Read the model definition and answer for the solid it produces. Units are mm, in the model's axes. A direction names the side the tool comes from. Round coordinates to 2 decimals unless told otherwise and drop trailing zeros. Loops run counter-clockwise (first coordinate to the right, second up) from the corner with the lowest first, then second, coordinate; pieces in that order, holes last. Notation, with made-up numbers: (70.25, 61.5) - (108.25, 61.5) arc R22 ccw to (108.25, 71.5) - close; hole circle Ø6 at (67, -19.75). An arc over 180 degrees is marked (long way). Use CSV: the item, a comma, the result in double quotes. Start each with the question number.
1. Determine the mould class of faces 1 (the cylindrical face through (9.921, 10.235, 1.014)), 2 (the flat face through (0, 5, 1)), 3 (the cylindrical face through (19.963, 10.801, 0.986)) for opening direction Y: +Y half, -Y half, draft (parallel to the pull), parting line (faces both ways), or undercut.
2. Find section B-B (y = 5). Give the vertices of the cut face in (x, z), and give its area (3 significant figures).
3. Consider line 1 along Y through (x, z) = (5, 1); line 2 along X through (y, z) = (5.25, 0.45); line 3 along X through (y, z) = (21, 0.6). Determine where each line is inside the solid, lowest interval first.
4. Find section C-C (z = 1.3). Give the vertices of the cut face in (x, y).
5. Find section A-A (x = 5). Give the vertices of the cut face in (y, z), and give its area (3 significant figures).
6. Given pin 1 Ø4 at (x, y) = (29.5, 20.5) entering from -Z; pin 2 Ø1 at (x, z) = (30.5, 0.5) entering from -Y, each flat-ended and moving along its own axis, determine where each tip first touches the part or whether it passes through.
7. A tool of negligible diameter and unlimited length cuts with its end or side. For faces 4 (the flat face through (6, 10, 1)), 5 (the cylindrical face through (9.98, 0.056, 1.014)), from which of +Z, -Z, +X, -X, +Y, -Y can it reach the whole face along a straight path? Write none if from no direction.
8. Find section D-D (x = 12). Give the vertices of the cut face in (y, z), and give its area (3 significant figures).
from build123d import *

# Parameters (mm, degrees)
SKETCH_1_R      = 1.6
EXTRUDE_2_DEPTH = 2
FILLET_1_R      = 3


with BuildPart() as part:
    # ｽｹｯﾁ1 → ﾎﾞｽ - 押し出し2 (new body)
    with BuildSketch(Plane.XY):
        Polygon((10, 10), (29.091883092, 29.091883092), (36.162950904, 22.02081528), (17.071067812, 2.928932188), (10, 0), (0, 0), (0, 10), align=None)
        with Locations((5, 5)):
            Circle(SKETCH_1_R, mode=Mode.SUBTRACT)
        with Locations((29.091883092, 22.02081528)):
            Circle(SKETCH_1_R, mode=Mode.SUBTRACT)
        with Locations((18.485281374, 11.414213562)):
            Circle(SKETCH_1_R, mode=Mode.SUBTRACT)
    extrude(amount=EXTRUDE_2_DEPTH)

    # ﾌｨﾚｯﾄ1
    fillet_1_edges = [part.edges().sort_by_distance(p)[0] for p in [
        (0, 0, 1),
        (0, 10, 1),
        (10, 10, 1),
        (29.091883092, 29.091883092, 1),
        (36.162950904, 22.02081528, 1),
        (17.071067812, 2.928932188, 1),
        (10, 0, 1),
    ]]
    fillet(fillet_1_edges, radius=FILLET_1_R)


solid = part.part
Filled sheet:
1,face 1,"+Y half"
1,face 2,"draft"
1,face 3,"undercut"
2,outline,"(0, 0) - (3.4, 0) - (3.4, 2) - (0, 2) - close; (6.6, 0) - (19.14, 0) - (19.14, 2) - (6.6, 2) - close"
2,area,"31.9 mm²"
3,line 1,"y = 0 to 3.4, 6.6 to 10"
3,line 2,"x = 0 to 3.42, 6.58 to 19.39"
3,line 3,"x = 21 to 27.86, 30.32 to 34.74"
4,outline,"(0, 3) arc R3 ccw to (3, 0) - (9.4, 0) arc R3 ccw to (10.55, 0.23) - (16.52, 2.7) arc R3 ccw to (17.49, 3.35) - (34.04, 19.9) arc R3 ccw to (34.04, 24.14) - (31.21, 26.97) arc R3 ccw to (26.97, 26.97) - (10.88, 10.88) arc R3 cw to (8.76, 10) - (3, 10) arc R3 ccw to (0, 7) - close; hole circle Ø3.2 at (5, 5); hole circle Ø3.2 at (18.49, 11.41); hole circle Ø3.2 at (29.09, 22.02)"
5,outline,"(0, 0) - (3.4, 0) - (3.4, 2) - (0, 2) - close; (6.6, 0) - (10, 0) - (10, 2) - (6.6, 2) - close"
5,area,"13.6 mm²"
6,pin 1,"stops at z = 0"
6,pin 2,"stops at y = 15.86"
7,face 4,"+Z, -Z, -X, +Y"
7,face 5,"+Z, -Z, +X, -Y"
8,outline,"(0.83, 0) - (12, 0) - (12, 2) - (0.83, 2) - close"
8,area,"22.3 mm²"
